Work out the finished part from the listing and answer in its coordinate system (mm). Coordinates: 2 decimals unless noted, no trailing zeros. Loops run counter-clockwise (first coordinate to the right, second up) from the corner with the lowest first, then second, coordinate; pieces in that order, holes last.
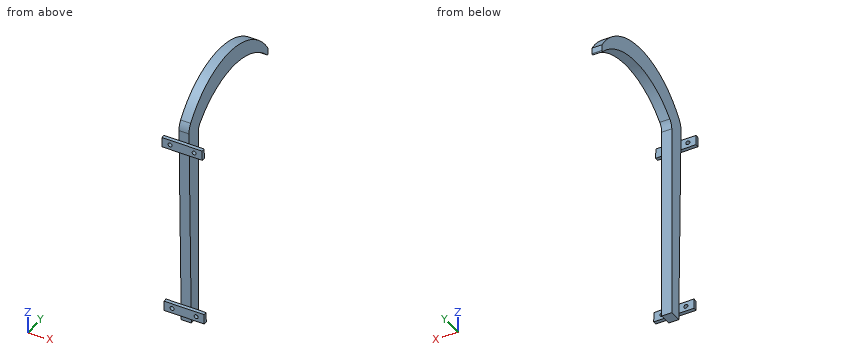
```python
from build123d import *

# Parameters (mm, degrees)
BOSS_EXTRUDE1_DEPTH = 15.875
SKETCH2_W           = 127
SKETCH2_H           = 31.75
SKETCH2_R           = 6.35
BOSS_EXTRUDE2_DEPTH = 11.176
FILLET1_R           = 2.54


with BuildPart() as part:
    # Sketch1 → Boss-Extrude1 (new, symmetric)
    with BuildSketch(Plane(origin=(0, 0, 0), x_dir=(0, 0, -1), z_dir=(1, 0, 0))):
        with BuildLine():
            Line((317.5, 0), (-302.771488663, 0))
            ThreePointArc((-302.771488663, 0), (-317.088938009, 2.792484593), (-329.307633721, 10.760596103))
            ThreePointArc((-329.307633721, 10.760596103), (-406.365714437, 197.196523766), (-323.223757211, 381))
            Line((-323.223757211, 381), (-348.623757211, 381))
            ThreePointArc((-348.623757211, 381), (-466.315322723, 172.429486078), (-358.266662239, -41.295689879))
            ThreePointArc((-358.266662239, -41.295689879), (-343.922523577, -48.296611465), (-328.11404497, -50.500975578))
            Line((-328.11404497, -50.500975578), (317.5, -38.1))
            Line((317.5, -38.1), (317.5, 0))
        make_face()
    extrude(amount=BOSS_EXTRUDE1_DEPTH, both=True)

    # Sketch2 → Boss-Extrude2 (add)
    # profile 1 of 2: a face of its own
    with BuildSketch(Plane(origin=(0, -44.182249353, -0.848654083), x_dir=(1, 0, 0), z_dir=(0, -0.9998155767735977, -0.019204490122845825))):
        with Locations((0, 279.4)):
            Rectangle(SKETCH2_W, SKETCH2_H)
        with Locations(Location((38.1, 279.4, 0), (0, 0, 270))):
            Circle(SKETCH2_R, mode=Mode.SUBTRACT)
        with Locations(Location((-38.1, 279.4, 0), (0, 0, 270))):
            Circle(SKETCH2_R, mode=Mode.SUBTRACT)
    # profile 2 of 2: a face of its own
    with BuildSketch(Plane(origin=(0, -44.182249353, -0.848654083), x_dir=(1, 0, 0), z_dir=(0, -0.9998155767735977, -0.019204490122845825))):
        with Locations((0, -279.4)):
            Rectangle(SKETCH2_W, SKETCH2_H)
        with Locations(Location((-38.1, -279.4, 0), (0, 0, 90))):
            Circle(SKETCH2_R, mode=Mode.SUBTRACT)
        with Locations(Location((38.1, -279.4, 0), (0, 0, 90))):
            Circle(SKETCH2_R, mode=Mode.SUBTRACT)
    extrude(amount=BOSS_EXTRUDE2_DEPTH)

    # Fillet1
    fillet1_edges = [part.edges().sort_by_distance(p)[0] for p in [
        (0, 381, 323.223757211),
    ]]
    fillet(fillet1_edges, radius=FILLET1_R)


solid = part.part
```
1. Straight lines are drawn through the part: probe 1 along Y at (x, z) = (8, -282.5); probe 2 along Y at (x, z) = (41.5, 269.5); probe 3 along Z at (x, y) = (3.5, 112). For each, find the intervals that lie inside material, in ascending order.
2. A cutting plane is placed at A-A, the plane x = -7. Give the vertices of the cut face in (y, z), then the cut area to 3 significant figures.
3. A cutting plane is placed at C-C, the plane y = 38. Give the vertices of the cut face in (x, z) (3 decimals).
4. A cutting plane is placed at B-B, the plane z = 312.5. Give the vertices of the cut face in (x, y) (3 decimals).
5. Each of these flat-tipped pins is pushed along its axis until it touches: P1, Ø3, axis at x = -16.5, z = 184.5, coming from the +Y side; P2, Ø5, axis at x = -5, z = 365, coming from the -Y side. Where does it stop, or does it pass through?
Answers below:
1. probe 1: y = -49.95 to 0
1. probe 2: y = -60.55 to -49.38
1. probe 3: z = 393.13 to 460.44
2. outline: (-61.03, 294.16) - (-60.42, 262.41) - (-49.24, 262.63) - (-39.12, -264.33) - (-50.3, -264.54) - (-49.69, -296.28) - (-38.51, -296.07) - (-38.1, -317.5) - (0, -317.5) - (0, 302.77) arc R38.1 cw to (10.76, 329.31) arc R254 cw to (376.62, 327.92) arc R2.54 ccw to (381, 329.67) - (381, 348.62) arc R254 ccw to (-41.3, 358.27) arc R50.8 ccw to (-50.5, 328.11) - (-49.85, 294.37) - close
2. area: 54,000 mm2
3. outline: (-15.875, 353.606) - (15.875, 353.606) - (15.875, 431.402) - (-15.875, 431.402) - close
4. outline: (-15.875, -50.201) - (15.875, -50.201) - (15.875, 1.263) - (-15.875, 1.263) - close
5. P1: stops at y = 0
5. P2: stops at y = -38.26
